```python
from build123d import *

# Parameters (mm, degrees)
SKETCH_1_W                   = 43
SKETCH_1_H                   = 170
EXTRUDE_296_DEPTH            = 7
SKETCH_2_W                   = 3
SKETCH_2_H                   = 170
EXTRUDE_513_DEPTH            = 3
HOLE_WIZARD_M5_2_D           = 5.5
HOLE_WIZARD_M5_2_CSINK_D     = 11.2
HOLE_WIZARD_M5_2_CSINK_ANGLE = 90
SKETCH_9_W                   = 183
SKETCH_9_H                   = 10
EXTRUDE_1613_DEPTH           = 170
SKETCH_10_W                  = 183
SKETCH_10_H                  = 10
EXTRUDE_1772_DEPTH           = 7
EXTRUDE_3_DEPTH              = 10
EXTRUDE_3_DEPTH_BACK         = 10
CUT_EXTRUDE_1_DEPTH          = 258.239674234
MIRROR_2_COPY_1_DEPTH        = 258.239674234
CUT_EXTRUDE_2_DEPTH          = 10
MIRROR_3_COPY_1_DEPTH        = 258.239674234
MIRROR_3_COPY_2_DEPTH        = 258.239674234
MIRROR_3_COPY_3_DEPTH        = 258.239674234


with BuildPart() as part:
    # 草图1 → Extrude 296 (new body)
    with BuildSketch(Plane.XY):
        Rectangle(SKETCH_1_W, SKETCH_1_H)
    extrude(amount=EXTRUDE_296_DEPTH)

    # 草图2 → Extrude 513 (add)
    with BuildSketch(Plane.XY.offset(7)):
        Rectangle(SKETCH_2_W, SKETCH_2_H)
    extrude(amount=EXTRUDE_513_DEPTH)

    # M5*2 沉头孔 (through all)
    with Locations(Plane(origin=(0, 0, 0), x_dir=(-1, 0, 0), z_dir=(0, 0, -1))):
        with Locations((0, 7), (0, -48)):
            CounterSinkHole(HOLE_WIZARD_M5_2_D / 2, HOLE_WIZARD_M5_2_CSINK_D / 2, counter_sink_angle=HOLE_WIZARD_M5_2_CSINK_ANGLE)

    # 草图9 → Extrude 1613 (add)
    with BuildSketch(Plane(origin=(0, 0, 0), x_dir=(-1, 0, 0), z_dir=(0, 0, -1))):
        with Locations((0, 80)):
            Rectangle(SKETCH_9_W, SKETCH_9_H)
    extrude(amount=EXTRUDE_1613_DEPTH)

    # 草图10 → Extrude 1772 (add)
    with BuildSketch(Plane.XY):
        with Locations((0, 80)):
            Rectangle(SKETCH_10_W, SKETCH_10_H)
    extrude(amount=EXTRUDE_1772_DEPTH)

    # 草图11 → 凸台-拉伸3 (add, two sides: drawn at the far end of the back side and taken through both)
    with BuildSketch(Plane(origin=(0, 0, 0), x_dir=(0, 0, -1), z_dir=(1, 0, 0)).offset(-EXTRUDE_3_DEPTH_BACK)):
        Polygon((0, 74.965878979), (0, 24.965878979), (120, 74.965878979), align=None)
    extrude(amount=EXTRUDE_3_DEPTH + EXTRUDE_3_DEPTH_BACK)

    # 草图12 → 切除-拉伸1 (cut, through all)
    with BuildSketch(Plane(origin=(0, 85, 0), x_dir=(1, 0, 0), z_dir=(0, 1, 0))):
        with BuildLine():
            Line((-74, 160), (-74, 140))
            ThreePointArc((-74, 140), (-77.5, 136.5), (-81, 140))
            Line((-81, 140), (-81, 160))
            ThreePointArc((-81, 160), (-77.5, 163.5), (-74, 160))
        make_face()
    cut_extrude_1 = extrude(amount=-CUT_EXTRUDE_1_DEPTH, mode=Mode.SUBTRACT)

    # 镜向1: 切除-拉伸1 across plane
    add(cut_extrude_1.mirror(Plane.XY.offset(-99.5)), mode=Mode.SUBTRACT)

    # 镜向2: 切除-拉伸1 across plane
    add(cut_extrude_1.mirror(Plane.ZY.offset(46.5)), mode=Mode.SUBTRACT)

    # 镜向2 copy 1 sketch → 镜向2 copy 1 (cut, through all)
    with BuildSketch(Plane(origin=(-93, 85, -199), x_dir=(-1, 0, 0), z_dir=(0, 1, 0))):
        with BuildLine():
            Line((-74, 160), (-74, 140))
            ThreePointArc((-74, 140), (-77.5, 136.5), (-81, 140))
            Line((-81, 140), (-81, 160))
            ThreePointArc((-81, 160), (-77.5, 163.5), (-74, 160))
        make_face()
    extrude(amount=-MIRROR_2_COPY_1_DEPTH, mode=Mode.SUBTRACT)

    # 草图13 → 切除-拉伸2 (cut)
    with BuildSketch(Plane(origin=(0, 85, 0), x_dir=(1, 0, 0), z_dir=(0, 1, 0))):
        Polygon((-91.5, -7), (-21.5, -7), (-91.5, 23), align=None)
    cut_extrude_2 = extrude(amount=-CUT_EXTRUDE_2_DEPTH, mode=Mode.SUBTRACT)

    # 镜向3: 切除-拉伸1, 切除-拉伸2 across plane
    add(cut_extrude_1.mirror(Plane(origin=(0, 0, 0), x_dir=(0, 0, 1), z_dir=(1, 0, 0))), mode=Mode.SUBTRACT)
    add(cut_extrude_2.mirror(Plane(origin=(0, 0, 0), x_dir=(0, 0, 1), z_dir=(1, 0, 0))), mode=Mode.SUBTRACT)

    # 镜向3 copy 1 sketch → 镜向3 copy 1 (cut, through all)
    with BuildSketch(Plane(origin=(0, 85, -199), x_dir=(-1, 0, 0), z_dir=(0, 1, 0))):
        with BuildLine():
            Line((-74, 160), (-74, 140))
            ThreePointArc((-74, 140), (-77.5, 136.5), (-81, 140))
            Line((-81, 140), (-81, 160))
            ThreePointArc((-81, 160), (-77.5, 163.5), (-74, 160))
        make_face()
    extrude(amount=-MIRROR_3_COPY_1_DEPTH, mode=Mode.SUBTRACT)

    # 镜向3 copy 2 sketch → 镜向3 copy 2 (cut, through all)
    with BuildSketch(Plane(origin=(93, 85, 0), x_dir=(1, 0, 0), z_dir=(0, 1, 0))):
        with BuildLine():
            Line((-74, 160), (-74, 140))
            ThreePointArc((-74, 140), (-77.5, 136.5), (-81, 140))
            Line((-81, 140), (-81, 160))
            ThreePointArc((-81, 160), (-77.5, 163.5), (-74, 160))
        make_face()
    extrude(amount=-MIRROR_3_COPY_2_DEPTH, mode=Mode.SUBTRACT)

    # 镜向3 copy 3 sketch → 镜向3 copy 3 (cut, through all)
    with BuildSketch(Plane(origin=(93, 85, -199), x_dir=(1, 0, 0), z_dir=(0, 1, 0))):
        with BuildLine():
            Line((-74, -160), (-74, -140))
            ThreePointArc((-74, -140), (-77.5, -136.5), (-81, -140))
            Line((-81, -140), (-81, -160))
            ThreePointArc((-81, -160), (-77.5, -163.5), (-74, -160))
        make_face()
    extrude(amount=-MIRROR_3_COPY_3_DEPTH, mode=Mode.SUBTRACT)


solid = part.part
```
Build history of the part. All positions in model axes, mm. A direction names the side the tool comes from. Give positions to 0.01 mm unless a question says otherwise; leave off trailing zeros. Order: outer loops, then holes, each group sorted by start corner. A loop starts at its lowest first (then second) coordinate and runs counter-clockwise, first axis right, second up. Notation, with made-up numbers: M 1.5,-35.5 L 6.5,-35.5 A37 ccw 6.5,2.5 Z; hole C 49,-7 d8. An arc over 180 degrees is marked long. Write item = value, one per line. Start each with the question number.
(1) Slice it at A-A on x = 15.5. Write the cut outline in (y, z).
(2) Pin check, flat tips, straight feed: pin 1 Ø6 at (x, y) = (18.5, -56.5) entering from -Z; pin 2 Ø2 at (y, z) = (-25, 5) entering from -X; pin 3 Ø0.9 at (y, z) = (-26, 9) entering from +X. Stop position of each tip, or through.
(3) Probe L1, parallel to Y at x = 0, z = 5.25; L2, parallel to X at y = 7, z = 5.25; L3, parallel to Z at x = 9, y = -5.5. List the from-to ranges inside material, lowest first. Write a range as [from, to].
(4) Which spindle directions (+Z, -Z, +X, -X, +Y, -Y) get a long thin tool onto all of the face, cutting with end or side? Do faces 4 (the flat face through (-1, 85, -81)), 5 (the flat face through (-81, 80, -150)). Say none if no direction does.
(5) Two-plate mould, pull along X, no slides. Class faces 1 (the flat face through (-56.01, 80.07, -7.79)), 2 (the flat face through (-0.14, 49.616, -59.16)), 3 (the cylindrical face through (77.4, 80.1, -136.5)): released by +X, released by -X, zero draft, split by the parting line, or undercut.
(6) Slice it at D-D on z = -51. Write the cut outline in (x, y).
(7) Slice it at B-B on z = -72. Write the cut outline in (x, y), plus the area to 3 significant figures.
(8) Slice it at C-C on y = -21.5. Write the cut outline in (x, z).
Responses:
q1.outline = M -85,0 L 75,0 L 75,-35.5 L 85,-35.5 L 85,7 L -85,7 Z; M 75,-170 L 85,-170 L 85,-163.5 L 75,-163.5 Z; M 75,-136.5 L 85,-136.5 L 85,-62.5 L 75,-62.5 Z
q2.pin_1 = 0
q2.pin_2 = -21.5
q2.pin_3 = 1.5
q3.L1 = [-85, -50.75], [-45.25, 4.25], [9.75, 85]
q3.L2 = [-21.5, -2.75], [2.75, 21.5]
q3.L3 = [0, 7]
q4.face_4 = +Z, -Z, +X, -X, +Y
q4.face_5 = +Y, -Y
q5.face_1 = released by -X
q5.face_2 = zero draft
q5.face_3 = undercut
q6.outline = M -91.5,75 L -81,75 L -81,85 L -91.5,85 Z; M -74,75 L -19,75 L -19,85 L -74,85 Z; M -12,75 L 12,75 L 12,85 L -12,85 Z; M -10,46.22 L 10,46.22 L 10,74.97 L -10,74.97 Z; M 19,75 L 74,75 L 74,85 L 19,85 Z; M 81,75 L 91.5,75 L 91.5,85 L 81,85 Z
q7.outline = M -91.5,75 L 91.5,75 L 91.5,85 L -91.5,85 Z; M -10,54.97 L 10,54.97 L 10,74.97 L -10,74.97 Z
q7.area = 2,230 mm2
q8.outline = M -21.5,0 L 21.5,0 L 21.5,7 L 1.5,7 L 1.5,10 L -1.5,10 L -1.5,7 L -21.5,7 Z
